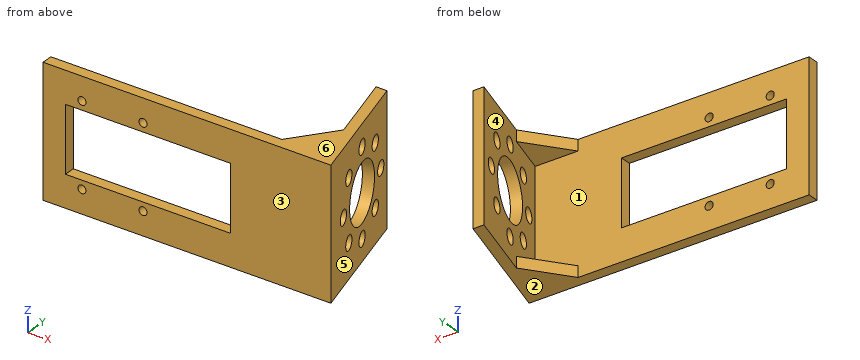
```python
from build123d import *

# Parameters (mm, degrees)
BOSS_EXTRUDE1_DEPTH = 57.15
BOSS_EXTRUDE2_DEPTH = 4.826
CUT_EXTRUDE1_REACH  = 124.673
SKETCH9_R           = 12.7
SKETCH11_R          = 3.175
CUT_EXTRUDE2_DEPTH  = 4.661558
CIRPATTERN1_COUNT   = 8
SKETCH12_R          = 1.778
SKETCH12_W          = 72.86244
SKETCH12_H          = 28.956
CUT_EXTRUDE4_DEPTH  = 5.826


with BuildPart() as part:
    # Sketch3 → Boss-Extrude1 (new body)
    with BuildSketch(Plane.XY):
        Polygon((-49.78, 0), (77.22, 0), (62.428491572, 55.202660972), (57.602491572, 55.202660972), (71.100877197, 4.826), (-49.78, 4.826), align=None)
    extrude(amount=BOSS_EXTRUDE1_DEPTH)

    # Sketch5 → Boss-Extrude2 (add)
    with BuildSketch(Plane.XY.offset(57.15)):
        Polygon((52.148255035, 4.826), (71.100877197, 4.826), (66.170374388, 23.226886991), align=None)
    boss_extrude2 = extrude(amount=-BOSS_EXTRUDE2_DEPTH)

    # Mirror1: Boss-Extrude2 across plane
    add(boss_extrude2.mirror(Plane(origin=(0, 0, 28.575), x_dir=(1, 0, 0), z_dir=(0, 0, -1))))

    # Sketch9 → Cut-Extrude1 (cut, up to next)
    with BuildSketch(Plane(origin=(72.04724084, 19.305, 0), x_dir=(0, 0, -1), z_dir=(0.965925826, 0.258819045, 0)), mode=Mode.PRIVATE) as cut_extrude1_sk1:
        with Locations((-28.575, 11.763993337)):
            Circle(SKETCH9_R)
    cut_extrude1_tool1 = extrude(cut_extrude1_sk1.sketch, amount=-CUT_EXTRUDE1_REACH, mode=Mode.PRIVATE) & part.part
    add(cut_extrude1_tool1.solids().sort_by_distance((69.002495, 30.668145, 28.575))[0], mode=Mode.SUBTRACT)

    # Sketch11 → Cut-Extrude2 (cut)
    with BuildSketch(Plane(origin=(72.04724084, 19.305, 0), x_dir=(0, 0, -1), z_dir=(0.965925826, 0.258819045, 0))):
        with Locations((-28.575, 30.813993337)):
            Circle(SKETCH11_R)
    cut_extrude2 = extrude(amount=-CUT_EXTRUDE2_DEPTH, mode=Mode.SUBTRACT)

    # CirPattern1: Cut-Extrude2 ×8 about axis
    cirpattern1_axis = Axis((-3.044745522, 11.363144985, 28.575), (0.965925826, 0.258819045, 0))
    for i in range(1, CIRPATTERN1_COUNT):
        add(cut_extrude2.rotate(cirpattern1_axis, i * 360 / CIRPATTERN1_COUNT), mode=Mode.SUBTRACT)

    # Sketch12 → Cut-Extrude4 (cut, through all)
    with BuildSketch(Plane(origin=(0, 4.826, 0), x_dir=(1, 0, 0), z_dir=(0, 1, 0))):
        with Locations((-32.595884, -46.863)):
            Circle(SKETCH12_R)
        with Locations((-5.65512, -46.863)):
            Circle(SKETCH12_R)
        with Locations((-3.44278, -28.575)):
            Rectangle(SKETCH12_W, SKETCH12_H)
    cut_extrude4 = extrude(amount=-CUT_EXTRUDE4_DEPTH, mode=Mode.SUBTRACT)

    # Mirror4: Cut-Extrude4 across plane
    add(cut_extrude4.mirror(Plane(origin=(0, 0, 28.575), x_dir=(1, 0, 0), z_dir=(0, 0, -1))), mode=Mode.SUBTRACT)


solid = part.part
```
The listing builds one solid part. Answer for the finished solid, in the listing's coordinates (mm). Face numbers are marked on the shaded views. A direction names the side the tool comes from. Give positions to 0.01 mm unless a question says otherwise; leave off trailing zeros. Write each loop counter-clockwise with the first axis right and the second up, starting at its lowest first coordinate (ties: lowest second). Pieces come first, ordered by that corner, then holes. Notation, with made-up numbers: (79.25, -35) - (134.25, -35) arc R15 cw to (134.25, -30) - close; hole circle Ø4 at (69, -12.75). An arc over 180 degrees is marked (long way). Use one line per item in the form item = value. Start each with the question number.
1) Find section C-C on x = 38. Determine the outline of the cut face in (y, z).
2) Consider line 1 along Y through (x, z) = (-41, 41); line 2 along X through (y, z) = (50, 32); line 3 along X through (y, z) = (46, 48.5). Determine where each line is inside the solid, lowest interval first. Write a range as from..to.
3) Flat-ended cylindrical pins translate along their axes: pin 1 Ø12 at (y, z) = (12.5, 28.5) entering from -X; pin 2 Ø1.5 at (y, z) = (45.5, 43) entering from -X; pin 3 Ø1 at (y, z) = (6.5, 40) entering from +X. Find the tip coordinate at first contact, or state that the pin passes through.
4) A tool of negligible diameter and unlimited length cuts with its end or side. For the marked faces 1 and 2, from which of +Z, -Z, +X, -X, +Y, -Y can it reach the whole face along a straight path? Write none if from no direction.
5) Find section B-B on z = 24. Determine the outline of the cut face in (x, y).
6) Find section A-A on x = 6. Determine the outline of the cut face in (y, z), plus the area to 3 significant figures.
7) The mould has two halves that part along Y. Classify the marked faces 3, 4, 5 and 6: pulls with the +Y half, pulls with the -Y half, needs draft (parallel to the pull), parting line crosses it, or undercut.
Geometry results:
q1.outline = (0, 0) - (4.83, 0) - (4.83, 57.15) - (0, 57.15) - close
q2.line_1 = 0..4.83
q2.line_2 = 59..63.82
q2.line_3 = 60.07..64.89
q3.pin_1 = 67.68
q3.pin_2 = 60
q3.pin_3 = 75.61
q4.face_1 = -X
q4.face_2 = -Z, +X, -X, +Y, -Y
q5.outline = (-49.78, 0) - (-39.87, 0) - (-39.87, 4.83) - (-49.78, 4.83) - close; (32.99, 0) - (77.22, 0) - (72.07, 19.22) - (67.57, 18.02) - (71.1, 4.83) - (32.99, 4.83) - close; (57.6, 55.2) - (61.43, 40.91) - (65.94, 42.11) - (62.43, 55.2) - close
q6.outline = (0, 0) - (4.83, 0) - (4.83, 14.1) - (0, 14.1) - close; (0, 43.05) - (4.83, 43.05) - (4.83, 57.15) - (0, 57.15) - close
q6.area = 136 mm2
q7.face_3 = pulls with the -Y half
q7.face_4 = undercut
q7.face_5 = pulls with the +Y half
q7.face_6 = needs draft
